Part model, mm, in its own coordinate system. Face numbers are marked on the shaded views. A direction names the side the tool comes from. Coordinates: 2 decimals unless noted, no trailing zeros. Order: outer loops, then holes, each group sorted by start corner. A loop starts at its lowest first (then second) coordinate and runs counter-clockwise, first axis right, second up. Notation, with made-up numbers: M -20.5,-33 L -12.5,-33 A19 cw -12.5,-29 Z; hole C 17.25,10.5 d4. An arc over 180 degrees is marked long. Write item = value, one per line. Start each with the question number.
from build123d import *

# Parameters (mm, degrees)
SKETCH_1_R          = 5
EXTRUDE_1_DEPTH     = 10
SKETCH_2_W          = 15
SKETCH_2_H          = 12
EXTRUDE_2_DEPTH     = 2
SKETCH_4_R          = 3
CUT_EXTRUDE_1_DEPTH = 16.370426149
SKETCH_5_W          = 3
SKETCH_5_H          = 12
EXTRUDE_3_DEPTH     = 20
SKETCH_6_OUTSIDE_W  = 21.464
SKETCH_6_OUTSIDE_H  = 41.464
CUT_EXTRUDE_2_DEPTH = 36.846896658
SKETCH_7_R          = 3
CUT_EXTRUDE_3_DEPTH = 36.809255992


with BuildPart() as part:
    # 草图1 → 凸台-拉伸1 (new body)
    with BuildSketch(Plane(origin=(0, 0, 0), x_dir=(1, 0, 0), z_dir=(0, 1, 0))):
        with Locations(Location((0, 0, 0), (0, 0, 270))):
            Circle(SKETCH_1_R)
    extrude(amount=EXTRUDE_1_DEPTH)

    # 草图2 → 凸台-拉伸2 (add)
    with BuildSketch(Plane(origin=(0, 10, 0), x_dir=(1, 0, 0), z_dir=(0, 1, 0))):
        Rectangle(SKETCH_2_W, SKETCH_2_H)
    extrude(amount=EXTRUDE_2_DEPTH)

    # 草图4 → 切除-拉伸1 (cut, through all)
    with BuildSketch(Plane(origin=(0, 0, 0), x_dir=(-1, 0, 0), z_dir=(0, -1, 0))):
        with Locations(Location((0, 0, 0), (0, 0, 90))):
            Circle(SKETCH_4_R)
    extrude(amount=-CUT_EXTRUDE_1_DEPTH, mode=Mode.SUBTRACT)

    # 草图5 → 凸台-拉伸3 (add)
    with BuildSketch(Plane(origin=(0, 12, 0), x_dir=(1, 0, 0), z_dir=(0, 1, 0))):
        with Locations((-6, 0)):
            Rectangle(SKETCH_5_W, SKETCH_5_H)
        with Locations((6, 0)):
            Rectangle(SKETCH_5_W, SKETCH_5_H)
    extrude(amount=EXTRUDE_3_DEPTH)

    # 草图6 outside → 切除-拉伸2 (cut, through all)
    with BuildSketch(Plane.ZY.offset(7.5)):
        with Locations((0, 16)):
            Rectangle(SKETCH_6_OUTSIDE_W, SKETCH_6_OUTSIDE_H)
        with BuildLine():
            Line((-6, -1.626301301), (-6, 25.957828691))
            ThreePointArc((-6, 25.957828691), (0, 31.957828691), (6, 25.957828691))
            Line((6, 25.957828691), (6, -1.626301301))
            ThreePointArc((6, -1.626301301), (0, -7.626301301), (-6, -1.626301301))
        make_face(mode=Mode.SUBTRACT)
    extrude(amount=-CUT_EXTRUDE_2_DEPTH, mode=Mode.SUBTRACT)

    # 草图7 → 切除-拉伸3 (cut, through all)
    with BuildSketch(Plane(origin=(7.5, 0, 0), x_dir=(0, 0, -1), z_dir=(1, 0, 0))):
        with Locations((0, 25.957828691)):
            Circle(SKETCH_7_R)
    extrude(amount=-CUT_EXTRUDE_3_DEPTH, mode=Mode.SUBTRACT)


solid = part.part
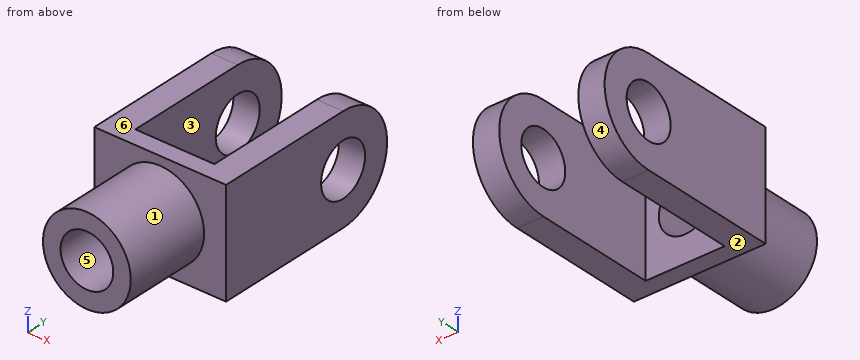
Item 1: 3-axis set-ups, long thin cutter, end or side, ignore diameter. For the marked faces 1, 2 and 3: which of +Z, -Z, +X, -X, +Y, -Y reach the whole face in a straight line?
Item 2: Wall check: line 1 along X through (y, z) = (27, -3.75); line 2 along Y through (x, z) = (-5.9, 0); line 3 along Y through (x, z) = (1.5, 5.75). Give the ranges that are in metal, low to high. Write a range as [from, to].
Item 3: Cut at B-B, the plane z = 0. Write the cut outline in (x, y).
Item 4: Cut at C-C, the plane x = 6.75. Write the cut outline in (y, z).
Item 5: Cut at A-A, the plane x = 0. Write the cut outline in (y, z).
Item 6: Cut at D-D, the plane y = 11.5. Write the cut outline in (x, z).
Item 7: Flat gauge pins, fed straight in: pin 1 (4.5 mm diameter, centred on x = 1, z = -2.5, fed in from +Y); pin 2 (1.5 mm diameter, centred on y = 4, z = 4, fed in from +X). Where does each tip first touch, or does it go through?
Item 8: Pull direction Z, two halves, no side cores. Call the marked faces 4, 5 and 6: pulls with the +Z half, pulls with the -Z half, needs draft (parallel to the pull), parting line crosses it, or undercut.
Filled sheet:
q1.face_1 = -Y
q1.face_2 = -Z, +X, -X, +Y, -Y
q1.face_3 = +Z, -Z, +Y
q2.line_1 = [-7.5, -4.5], [4.5, 7.5]
q2.line_2 = [10, 22.96], [28.96, 31.96]
q2.line_3 = [10, 12]
q3.outline = M -7.5,10 L -5,10 L -5,0 L -3,0 L -3,12 L -4.5,12 L -4.5,22.96 L -7.5,22.96 Z; M -7.5,28.96 L -4.5,28.96 L -4.5,31.96 L -7.5,31.96 Z; M 3,0 L 5,0 L 5,10 L 7.5,10 L 7.5,22.96 L 4.5,22.96 L 4.5,12 L 3,12 Z; M 4.5,28.96 L 7.5,28.96 L 7.5,31.96 L 4.5,31.96 Z
q4.outline = M 10,-6 L 25.96,-6 A6 ccw 25.96,6 L 10,6 Z; hole C 25.96,0 d6
q5.outline = M 0,-5 L 10,-5 L 10,-6 L 12,-6 L 12,-3 L 0,-3 Z; M 0,3 L 12,3 L 12,6 L 10,6 L 10,5 L 0,5 Z
q6.outline = M -7.5,-6 L 7.5,-6 L 7.5,6 L -7.5,6 Z; hole C 0,0 d6
q7.pin_1 = 12
q7.pin_2 = 3.8
q8.face_4 = parting line crosses it
q8.face_5 = undercut
q8.face_6 = pulls with the +Z half
